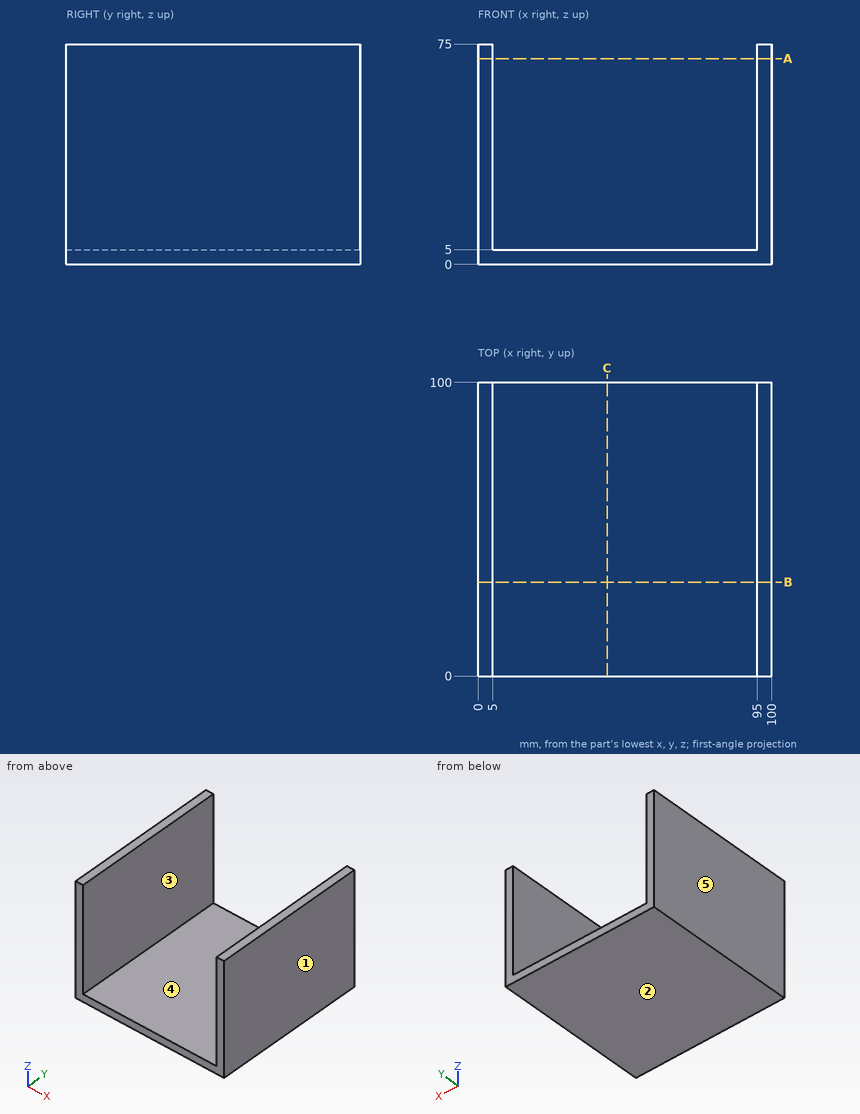
Input: dimensioned drawing with shaded views. Units: mm. Origin: part minimum x, y, z. A direction names the side the tool comes from. Give positions to 0.01 mm unless a question says otherwise; leave off trailing zeros. Loops run counter-clockwise (first coordinate to the right, second up) from the corner with the lowest first, then second, coordinate; pieces in that order, holes last. Notation, with made-up numbers: M 5,27.25 L 54,27.25 A7 ccw 54,40.25 Z; hole C 75.5,11.5 d6. An arc over 180 degrees is marked long. Put each result on its own line as item: value.
1) Cut plane A-A, the plane z = 70. Return the cut outline in (x, y), plus the area to 3 significant figures.
Computed values:
outline: M 0,0 L 5,0 L 5,100 L 0,100 Z; M 95,0 L 100,0 L 100,100 L 95,100 Z
area: 1,000 mm^2
2) Material intervals for L1, parallel to X at y = 79.5, z = 44; L2, parallel to Z at x = 49, y = 95, sorted ascending. Write a range as from..to.
Computed values:
L1: x = 0..5, 95..100
L2: z = 0..5
3) Mould query, pull axis X, two halves, no side actions, for the marked faces 1, 2 and 3. Classes: released by +X, released by -X, zero draft, split by the parting line, or undercut.
Computed values:
face 1: released by +X
face 2: zero draft
face 3: undercut
4) Cut plane B-B, the plane y = 32. Return the cut outline in (x, z), plus the area to 3 significant figures.
Computed values:
outline: M 0,0 L 100,0 L 100,75 L 95,75 L 95,5 L 5,5 L 5,75 L 0,75 Z
area: 1,200 mm^2
5) Reachability of the marked faces 4 and 5 from +Z, -Z, +X, -X, +Y, -Y: full face, straight path, thin tool, end or side. Return the list, or none.
Computed values:
face 4: +Z, +Y, -Y
face 5: +Z, -Z, -X, +Y, -Y
6) First-contact query: P1, Ø5, axis at x = 85.5, y = 64.5, coming from the +Z side. Flat tip, straight axial feed; report the tip coordinate or a pass-through.
Computed values:
P1: stops at z = 5
7) Cut plane C-C, the plane x = 44. Return the cut outline in (y, z), plus the area to 3 significant figures.
Computed values:
outline: M 0,0 L 100,0 L 100,5 L 0,5 Z
area: 500 mm^2
